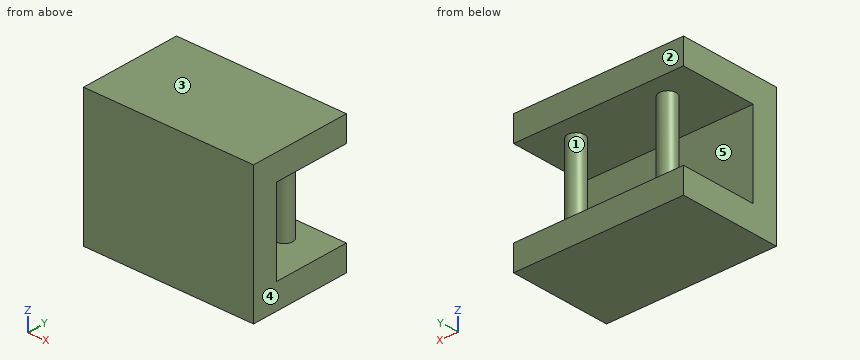
```python
from build123d import *

# Parameters (mm, degrees)
BOSS_EXTRUDE1_DEPTH = 100
SKETCH2_R           = 5
BOSS_EXTRUDE2_DEPTH = 50


with BuildPart() as part:
    # Sketch1 → Boss-Extrude1 (new body)
    with BuildSketch(Plane(origin=(0, 0, 0), x_dir=(0, 0, -1), z_dir=(1, 0, 0))):
        Polygon((0, 0), (0, 60), (15, 60), (15, 15), (65, 15), (65, 60), (80, 60), (80, 0), align=None)
    extrude(amount=BOSS_EXTRUDE1_DEPTH)

    # Sketch2 → Boss-Extrude2 (add)
    with BuildSketch(Plane(origin=(0, 0, -15), x_dir=(-1, 0, 0), z_dir=(0, 0, -1))):
        with Locations(Location((-77, 45, 0), (0, 0, 270))):
            Circle(SKETCH2_R)
        with Locations(Location((-23, 45, 0), (0, 0, 270))):
            Circle(SKETCH2_R)
    extrude(amount=BOSS_EXTRUDE2_DEPTH)


solid = part.part
```
Build history of the part. All positions in model axes, mm. Face numbers are marked on the shaded views. A direction names the side the tool comes from. Round coordinates to 2 decimals unless told otherwise and drop trailing zeros. Write each loop counter-clockwise with the first axis right and the second up, starting at its lowest first coordinate (ties: lowest second). Pieces come first, ordered by that corner, then holes. Notation, with made-up numbers: (-31.75, 58.5) -> (19.25, 58.5) arc R25 ccw to (19.25, 84.5) -> close; hole circle Ø9 at (24, 84). An arc over 180 degrees is marked (long way). Put each result on its own line as item: value.
Item 1: Slice it at A-A, the plane y = 28.5. Give the cut face in (x, z).
Here are the results:
outline: (0, -80) -> (100, -80) -> (100, -65) -> (0, -65) -> close; (0, -15) -> (100, -15) -> (100, 0) -> (0, 0) -> close
Item 2: Two-plate mould, pull along Z, no slides. Class the marked faces 3, 4 and 5: pulls with the +Z half, pulls with the -Z half, needs draft (parallel to the pull), parting line crosses it, or undercut.
Here are the results:
face 3: pulls with the +Z half
face 4: needs draft
face 5: undercut
Item 3: Slice it at C-C, the plane x = 23. Give the cut face in (y, z), plus the area to 3 significant figures.
Here are the results:
outline: (0, -80) -> (60, -80) -> (60, -65) -> (50, -65) -> (50, -15) -> (60, -15) -> (60, 0) -> (0, 0) -> close; hole (15, -65) -> (40, -65) -> (40, -15) -> (15, -15) -> close
area: 3,050 mm^2
Item 4: Flat gauge pins, fed straight in: P1, Ø13.5, axis at x = 50.5, y = 46.5, coming from the +Z side; P2, Ø4, axis at y = 47.5, z = -45, coming from the -X side; P3, Ø15, axis at x = 28.5, z = -35.5, coming from the +Y side. Where does each tip first touch, or does it go through?
Here are the results:
P1: stops at z = 0
P2: stops at x = 18.03
P3: stops at y = 50
Item 5: Wall check: probe 1 along Z at (x, y) = (75.5, 17.5); probe 2 along X at (y, z) = (44.5, -26); probe 3 along Y at (x, z) = (63, -30). Give the ranges that are in metal, low to high. Write a range as from..to.
Here are the results:
probe 1: z = -80..-65, -15..0
probe 2: x = 18.03..27.97, 72.03..81.97
probe 3: y = 0..15
Item 6: Slice it at D-D, the plane y = 45. Give the cut face in (x, z), plus the area to 3 significant figures.
Here are the results:
outline: (0, -80) -> (100, -80) -> (100, -65) -> (82, -65) -> (82, -15) -> (100, -15) -> (100, 0) -> (0, 0) -> (0, -15) -> (18, -15) -> (18, -65) -> (0, -65) -> close; hole (28, -65) -> (72, -65) -> (72, -15) -> (28, -15) -> close
area: 4,000 mm^2
Item 7: Tool access for the marked faces 1 and 2: list every direction of +Z, -Z, +X, -X, +Y, -Y with a clear straight run to the whole face (end or side of a thin tool).
Here are the results:
face 1: none
face 2: +Z, -Z, +X, -X, +Y
Item 8: Slice it at B-B, the plane z = -46. Give the cut face in (x, y), plus the area to 3 significant figures.
Here are the results:
outline: (0, 0) -> (100, 0) -> (100, 15) -> (0, 15) -> close; circle Ø10 at (23, 45); circle Ø10 at (77, 45)
area: 1,660 mm^2
